Study the drawing (mm; zero at the part's minimum x, y, z) and answer. Give positions to 0.01 mm unless a question says otherwise; leave off trailing zeros. One line per question, with ' | ' between items.
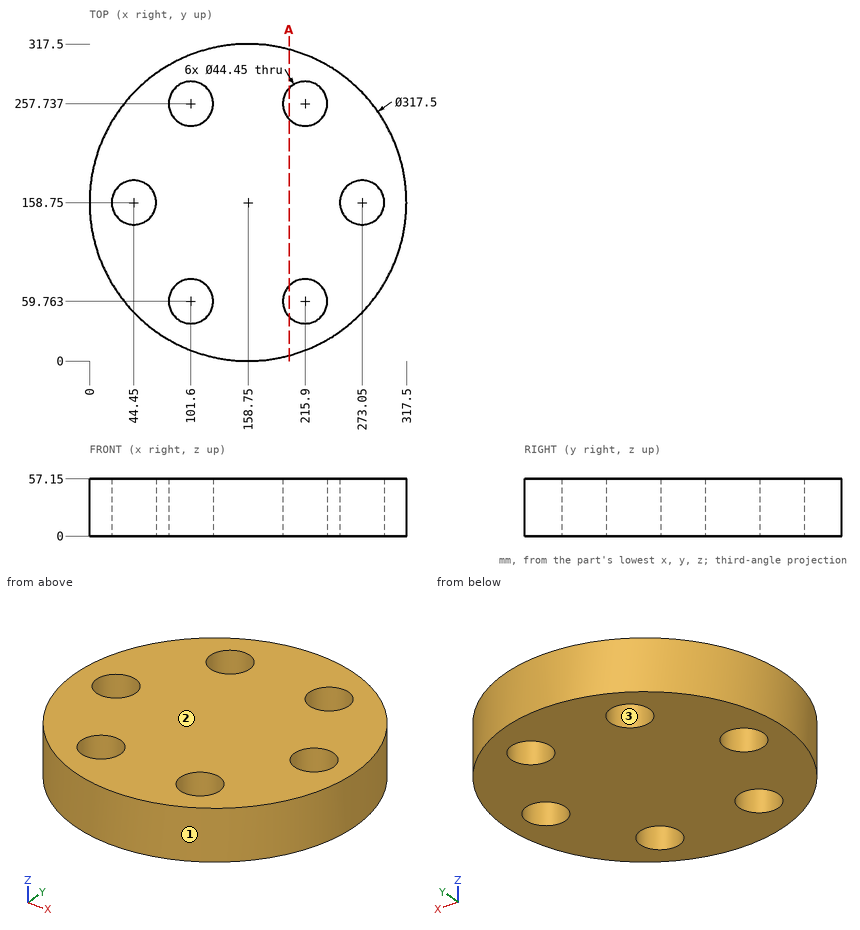
Item 1: Consider line 1 (X direction, y = 54, z = 31) (1 decimal); line 2 (X direction, y = 247, z = 19); line 3 (Y direction, x = 105, z = 41.5). Determine where each line is inside the solid, lowest interval first. Write a range as [from, to].
Answers below:
line 1: [39.5, 80.1], [123.1, 194.4], [237.4, 278] | line 2: [26.79, 82.14], [121.06, 196.44], [235.36, 290.71] | line 3: [9.38, 37.8], [81.73, 235.77], [279.7, 308.12]
Item 2: Find section A-A (x = 200). Count the separate pieces of the cut face and the enclosed holes in it, then the cut area to 3 significant figures.
Answers below:
separate pieces: 3 | enclosed holes: 0 | area: 14,000 mm²
Item 3: Determine the mould class of the marked faces 1, 2 and 3 for opening direction X: pulls with the +X half, pulls with the -X half, needs draft (parallel to the pull), parting line crosses it, or undercut.
Answers below:
face 1: parting line crosses it | face 2: needs draft | face 3: undercut
Item 4: Flat-ended cylindrical pins translate along their axes: pin 1 (5 mm diameter, centred on y = 230, z = 40, fed in from -X); pin 2 (5 mm diameter, centred on y = 200, z = 17, fed in from -X); pin 3 (6 mm diameter, centred on x = 228, z = 29.5, fed in from +Y) (1 decimal). Find the tip coordinate at first contact, or state that the pin passes through.
Answers below:
pin 1: x = 15.66 | pin 2: x = 4.8 | pin 3: y = 303
